Geometry: final body of the model. Coordinates: model frame, mm. Round coordinates to 2 decimals unless told otherwise and drop trailing zeros. Loops run counter-clockwise (first coordinate to the right, second up) from the corner with the lowest first, then second, coordinate; pieces in that order, holes last. Notation, with made-up numbers: M -6.5,46.5 L 52.5,46.5 A14 ccw 52.5,71.5 Z; hole C -20.75,54.5 d5. An arc over 180 degrees is marked long. Return JSON: item names as keys, results as strings.
from build123d import *

# Parameters (mm, degrees)
SKETCH1_R           = 5
SKETCH1_R_2         = 2
BOSS_EXTRUDE1_DEPTH = 2.5


with BuildPart() as part:
    # Sketch1 → Boss-Extrude1 (new, symmetric)
    with BuildSketch(Plane.XY):
        with BuildLine():
            Line((-63.5, 8), (63.5, 8))
            ThreePointArc((63.5, 8), (71.5, 0), (63.5, -8))
            Line((63.5, -8), (-63.5, -8))
            ThreePointArc((-63.5, -8), (-71.5, 0), (-63.5, 8))
        make_face()
        with Locations((-63.5, 0)):
            Circle(SKETCH1_R, mode=Mode.SUBTRACT)
        with Locations((63.5, 0)):
            Circle(SKETCH1_R, mode=Mode.SUBTRACT)
        Circle(SKETCH1_R_2, mode=Mode.SUBTRACT)
    extrude(amount=BOSS_EXTRUDE1_DEPTH, both=True)


solid = part.part
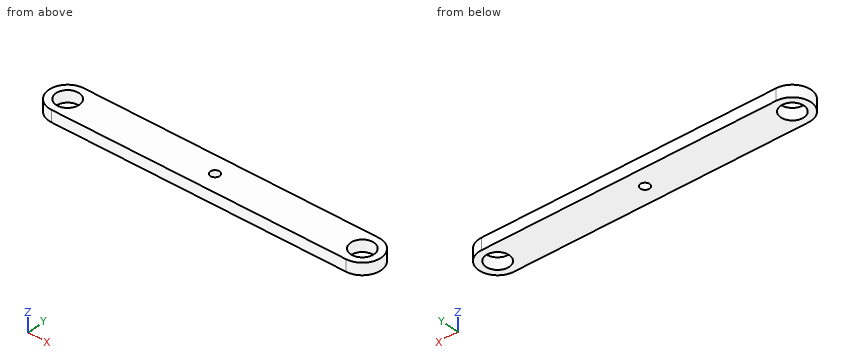
Q1. Section query A-A (x = 0). Output: boundary loops of the cut face in (y, z), plus the area to 3 significant figures.
Determined:
{"outline": "M -8,-2.5 L -2,-2.5 L -2,2.5 L -8,2.5 Z; M 2,-2.5 L 8,-2.5 L 8,2.5 L 2,2.5 Z", "area": "60.0 mm^2"}
Q2. Material intervals for L1, parallel to Y at x = -64, z = 1.5; L2, parallel to X at y = 1.75, z = -0.4; L3, parallel to X at y = -1.25, z = -1.15, sorted ascending.
Determined:
{"L1": "y = -7.98 to -4.97, 4.97 to 7.98", "L2": "x = -71.31 to -68.18, -58.82 to -0.97, 0.97 to 58.82, 68.18 to 71.31", "L3": "x = -71.4 to -68.34, -58.66 to -1.56, 1.56 to 58.66, 68.34 to 71.4"}
Q3. Section query C-C (z = 1.2). Output: boundary loops of the cut face in (x, y), plus the area to 3 significant figures.
Determined:
{"outline": "M -63.5,-8 L 63.5,-8 A8 ccw 63.5,8 L -63.5,8 A8 ccw Z; hole C -63.5,0 d10; hole C 0,0 d4; hole C 63.5,0 d10", "area": "2,060 mm^2"}
Q4. Section query B-B (y = 0). Output: boundary loops of the cut face in (x, z).
Determined:
{"outline": "M -71.5,-2.5 L -68.5,-2.5 L -68.5,2.5 L -71.5,2.5 Z; M -58.5,-2.5 L -2,-2.5 L -2,2.5 L -58.5,2.5 Z; M 2,-2.5 L 58.5,-2.5 L 58.5,2.5 L 2,2.5 Z; M 68.5,-2.5 L 71.5,-2.5 L 71.5,2.5 L 68.5,2.5 Z"}
Q5. Pin query (flat end, axial travel): pin 1 (3 mm diameter, centred on y = 6, z = -0.5, fed in from +X); pin 2 (1.5 mm diameter, centred on y = 1, z = 0.5, fed in from -X). Return the tip coordinate at first contact, or that it passes through.
Determined:
{"pin 1": "stops at x = 70.11", "pin 2": "stops at x = -71.5"}
